```python
from build123d import *

# Parameters (mm, degrees)
BOSS_EXTRUDE1_DEPTH      = 125
BOSS_EXTRUDE1_DEPTH_BACK = 75
SKETCH1_R                = 10
BOSS_EXTRUDE2_START      = 15
BOSS_EXTRUDE2_DEPTH      = 7.5
BODY_MOVE_COPY1_ANGLE    = 90
CUT_EXTRUDE1_DEPTH       = 4


with BuildPart() as part:
    # Sketch1 → Boss-Extrude1 (new, two sides: drawn at the far end of the back side and taken through both)
    with BuildSketch(Plane(origin=(0, 0, 0), x_dir=(0, 0, -1), z_dir=(1, 0, 0)).offset(-BOSS_EXTRUDE1_DEPTH_BACK)):
        Circle(SKETCH1_R)
    extrude(amount=BOSS_EXTRUDE1_DEPTH + BOSS_EXTRUDE1_DEPTH_BACK)

    # Sketch3 → Cut-Extrude1 (cut)
    with BuildSketch(Plane(origin=(0, 10, 0), x_dir=(1, 0, 0), z_dir=(0, 1, 0))):
        with BuildLine():
            Line((97, 4), (117, 4))
            ThreePointArc((117, 4), (121, 0), (117, -4))
            Line((117, -4), (97, -4))
            ThreePointArc((97, -4), (93, 0), (97, 4))
        make_face()
    extrude(amount=-CUT_EXTRUDE1_DEPTH, mode=Mode.SUBTRACT)


with BuildPart() as body_2:
    # Sketch2 → Boss-Extrude2 (new, symmetric)
    with BuildSketch(Plane(origin=(0, 0, 0), x_dir=(0, 0, -1), z_dir=(1, 0, 0)).offset(BOSS_EXTRUDE2_START)):
        with BuildLine():
            ThreePointArc((-4.867089568, 10.968657125), (-10.868088345, -5.087696504), (5.306226617, -10.763083159))
            ThreePointArc((5.306226617, -10.763083159), (10.673744978, -7.573594418), (15.479542802, -3.587694386))
            ThreePointArc((15.479542802, -3.587694386), (16.864464688, -1.143374761), (16.712672037, 1.661917746))
            ThreePointArc((16.712672037, 1.661917746), (7.958571112, 11.035699457), (-4.867089568, 10.968657125))
        make_face()
    extrude(amount=BOSS_EXTRUDE2_DEPTH, both=True)


with BuildPart() as body_3:
    # Mirror1: mirrored copy
    add(body_2.part.mirror(Plane(origin=(0, 0, 0), x_dir=(0, 0, 1), z_dir=(1, 0, 0))))


with BuildPart() as body_3_1:
    # Body-Move/Copy1: moved
    add(body_3.part.rotate(Axis((0, 0, 0), (-1, 0, 0)), BODY_MOVE_COPY1_ANGLE))


with BuildPart() as part_1:
    add(part.part)

    # Combine1: union body 3, body 2
    add(body_3_1.part)
    add(body_2.part)


solid = part_1.part
```
Check sheet for the modelled part. Datum: model origin and axes. Units: mm. A direction names the side the tool comes from. Give positions to 0.01 mm unless a question says otherwise; leave off trailing zeros. Write each loop counter-clockwise with the first axis right and the second up, starting at its lowest first coordinate (ties: lowest second). Pieces come first, ordered by that corner, then holes.
Item 1: Access from +Z, -Z, +X, -X, +Y, -Y to the whole of each face (thin tool, end or side, straight path). Record for faces 1 (the face through (-15.105, -10.602, 7.624)), 2 (the face through (7.5, 2, -10)), 3 (the face through (-22.5, -10, -2)), 4 (the face through (73.03, -9.76, 2.17)), 5 (the face through (107, 8, -4)).
Item 2: Cross-section at A-A (x = 99.5). Enter the section's corners in (y, z).
Item 3: Scan lines: L1, parallel to X at y = 8.5, z = -5.75; L2, parallel to X at y = -13.5, z = -3; L3, parallel to X at y = 7.75, z = 3.25. Record each from-to range of solid material in increasing order.
Item 4: Cross-section at B-B (z = 0). Enter the section's corners in (x, y), and give its area (3 significant figures).
Item 5: Draft check along X on faces 6 (the face through (107, 6, 0)), 7 (the face through (-7.5, -10, -2)), 8 (the face through (15.105, -7.624, -10.602)), 9 (the face through (-75, 0, 0)). Enter one of: released by +X, released by -X, zero draft, split by the parting line, or undercut.
Item 6: Gauge pin test, flat ends, axial feed: pin 1 (1 mm diameter, centred on y = 9.5, z = -6, fed in from +X); pin 2 (6.5 mm diameter, centred on x = 103.5, z = 0, fed in from +Y); pin 3 (3 mm diameter, centred on x = 42, y = -7.5, fed in from +Z). Record the tip position at first contact, or that the pin passes through.
Item 7: Cross-section at D-D (x = 69). Enter the section's corners in (y, z), and give its area (3 significant figures).
Item 8: Cross-section at C-C (y = 0). Enter the section's corners in (x, z).
Report:
1. face 1: +Z, +X, -X, -Y
1. face 2: none
1. face 3: -X
1. face 4: +X
1. face 5: +Y
2. outline: (6, -4) - (6, 4) - (9.17, 4) arc R10 ccw (long way) to (9.17, -4) - close
3. L1: x = -22.5 to -7.5, 7.5 to 22.5
3. L2: x = -22.5 to -7.5
3. L3: x = -75 to 94.67, 119.33 to 125
4. outline: (-75, -10) - (-22.5, -10) - (-22.5, -17) - (-7.5, -17) - (-7.5, -10) - (7.5, -10) - (7.5, -12) - (22.5, -12) - (22.5, -10) - (125, -10) - (125, 10) - (121, 10) - (121, 6) - (93, 6) - (93, 10) - (22.5, 10) - (22.5, 12.26) - (7.5, 12.26) - (7.5, 10) - (-7.5, 10) - (-7.5, 12) - (-22.5, 12) - (-22.5, 10) - (-75, 10) - close
4. area: 4,090 mm2
5. face 6: undercut
5. face 7: undercut
5. face 8: zero draft
5. face 9: released by -X
6. pin 1: stops at x = 22.5
6. pin 2: stops at y = 6
6. pin 3: stops at z = 8
7. outline: circle Ø20 at (0, 0)
7. area: 314 mm2
8. outline: (-75, -10) - (-22.5, -10) - (-22.5, -12.26) - (-7.5, -12.26) - (-7.5, -10) - (7.5, -10) - (7.5, -17) - (22.5, -17) - (22.5, -10) - (125, -10) - (125, 10) - (22.5, 10) - (22.5, 12) - (7.5, 12) - (7.5, 10) - (-7.5, 10) - (-7.5, 12) - (-22.5, 12) - (-22.5, 10) - (-75, 10) - close
